Design review of the part built by this model. Coordinates are the model's own, in mm. Coordinates: 2 decimals unless noted, no trailing zeros. Write each loop counter-clockwise with the first axis right and the second up, starting at its lowest first coordinate (ties: lowest second). Pieces come first, ordered by that corner, then holes.
Q1. Insertion check: pin 1 (0.8 mm diameter, centred on x = 0.5, y = -3, fed in from -Z); pin 2 (2.5 mm diameter, centred on y = 201.15, z = -46.03, fed in from +X). Each pin has a flat end and moves straight along its axis. Give the tip position at first contact, or say it passes through.
Q2. Take a section at A-A (y = 28). Give the boundary of the cut face in (x, z).
Q3. Take a section at C-C (z = -31.5). Give the boundary of the cut face in (x, y).
Q4. For probe 1 along Z at (x, y) = (1.1, -4); probe 2 along Z at (x, y) = (0.85, 39); probe 3 along Y at (x, z) = (0.8, -5), list the stretches that pass through material, from the lowest coordinate up.
Q5. Take a section at B-B (x = 1.15). Give the boundary of the cut face in (y, z) (1 decimal), and give its area (3 significant figures).
Autodesk Inventor part; units mm, degrees
ref_plane "YZ Plane" through (0, 0, 0) normal (1, 0, 0) x (0, 1, 0)
ref_plane "XZ Plane" through (0, 0, 0) normal (0, 1, 0) x (-1, 0, 0)
ref_plane "XY Plane" through (0, 0, 0) normal (0, 0, 1) x (1, 0, 0)
sketch "Sketch2" plane through (0, 0, 0) normal (1, 0, 0) x (0, 1, 0)
  line L0 (0, 4) -> (60, 4)
  line L1 (0, 0) -> (60, 0)
  line L2 (0, -61) -> (0, 14)
  line L3 (96.4802, -36) -> (98.4802, -26)
  line L4 (96.4802, -36) -> (110.2083, 32.6406)
  line L5 (0, 0) -> (103.6802, 0)
  line L6 (0, 0) -> (0, -10)
  line L7 (0, -10) -> (101.6802, -10)
  line L8 (0, 0) -> (0, -2.5)
  line L9 (0, -2.5) -> (-7, -2.5)
  line L10 (-7, -2.5) -> (-7, -7.5)
  line L11 (-7, -7.5) -> (0, -7.5)
  line L12 (0, -2.5) -> (-4, -2.5)
  line L13 (-4, -2.5) -> (-4, -5)
  circle A0 centre (-4, -5) radius 1.5
  line L14 (198.4235, -42.1847) -> (202.1158, -43.7232)
  line L15 (204.885, -44.877) -> (202.9619, -49.4924)
  line L16 (198.4235, -42.1847) -> (204.885, -44.877)
  line L17 (202.9619, -49.4924) -> (196.5004, -46.8001)
  circle A1 centre (201.1542, -46.0308) radius 1.5
  line L18 (199.385, -39.877) -> (195.5388, -49.1078)
  line L19 (199.385, -39.877) -> (144.0004, -16.8001)
  line L20 (195.5388, -49.1078) -> (101.6802, -10)
  line L21 (199.385, -39.877) -> (103.6802, 0)
  point P0 (0, -7.5)
  dimension "d10" = 70
  dimension "d11" = 10
  dimension "d12" = 2.5
  dimension "d13" = 7
  dimension "d14" = 5
  dimension "d15" = 4
  dimension "d16" = 2.5
  dimension "d17" = 3
extrude "Extrusion2" add sketch "Sketch2" along normal blind 1.5
properties part number "MotorSupport"
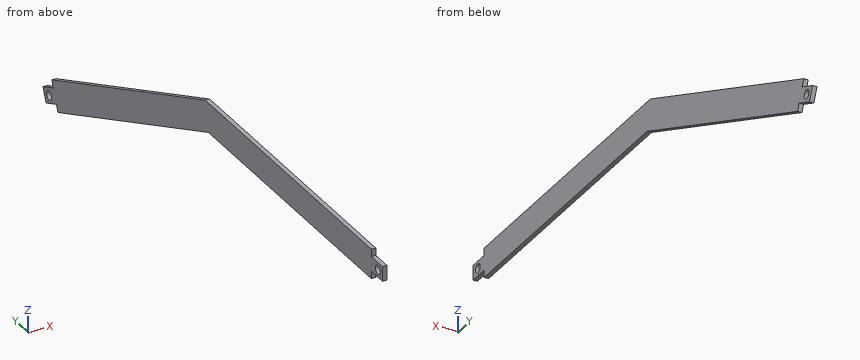
Response:
1. pin 1: stops at z = -7.5
1. pin 2: passes through
2. outline: (0, -10) - (1.5, -10) - (1.5, 0) - (0, 0) - close
3. outline: (0, 153.28) - (1.5, 153.28) - (1.5, 179.28) - (0, 179.28) - close
4. probe 1: z = -7.5 to -6.5, -3.5 to -2.5
4. probe 2: z = -10 to 0
4. probe 3: y = -7 to -5.5, -2.5 to 115.68
5. outline: (-7, -7.5) - (0, -7.5) - (0, -10) - (101.7, -10) - (195.5, -49.1) - (196.5, -46.8) - (203, -49.5) - (204.9, -44.9) - (202.1, -43.7) - (198.4, -42.2) - (199.4, -39.9) - (144, -16.8) - (103.7, 0) - (0, 0) - (0, -2.5) - (-7, -2.5) - close; hole circle Ø3 at (-4, -5); hole circle Ø3 at (201.2, -46)
5. area: 2,110 mm2
